Solid Edge part; units mm, degrees
sketch "Sketch1" plane through (0, 0, 0) normal (0, -1, 0) x (1, 0, 0)
  line L0 (-7.5, 10.5) -> (0, 10.5)
  line L1 (0, 10.5) -> (0, 2.95)
  line L2 (-7.5, 2.95) -> (0, 2.95)
  line L3 (-7.5, 10.5) -> (-7.5, 2.95)
  dimension "D1" = 7.5
revolve "RevolvedProtrusion1" add sketch "Sketch1" angle 360 about axis through (0, 0, 0) along (1, 0, 0)
sketch "Sketch2" plane through (-7.5, 0, 0) normal (-1, 0, 0) x (0, -1, 0)
  line L0 (2.9445, -5.1) -> (5.889, 0)
  line L1 (5.889, 0) -> (2.9445, 5.1)
  line L2 (2.9445, 5.1) -> (-2.9445, 5.1)
  line L3 (-2.9445, 5.1) -> (-5.889, 0)
  line L4 (-5.889, 0) -> (-2.9445, -5.1)
  line L5 (-2.9445, -5.1) -> (2.9445, -5.1)
extrude "Cutout1" cut sketch "Sketch2" against normal blind 4.5
chamfer "Fase_2" distance 0.5 angle 45 2 edges at (-7.5, 0, -10.5) (0, 0, -10.5)
hole "Bohrung_1" at (0, -8, 0) direction (-1, 0, 0) diameter 2.2 end up to next
hole "Hole1" at (0, 0, 8) direction (-1, 0, 0) diameter 2.2 end up to next
hole "Hole2" at (0, 0, -8) direction (-1, 0, 0) diameter 2.2 end up to next
hole "Hole3" at (0, 8, 0) direction (-1, 0, 0) diameter 2.2 end up to next
hole "Bohrung_5" at (0, -8, 0) direction (-1, 0, 0) diameter 5.5 depth 2
hole "Hole4" at (0, 0, 8) direction (-1, 0, 0) diameter 5.5 depth 2
hole "Hole5" at (0, 8, 0) direction (-1, 0, 0) diameter 5.5 depth 2
hole "Hole6" at (0, 0, -8) direction (-1, 0, 0) diameter 5.5 depth 2
Part model, mm, in its own coordinate system. A direction names the side the tool comes from. Coordinates: 2 decimals unless noted, no trailing zeros. Write each loop counter-clockwise with the first axis right and the second up, starting at its lowest first coordinate (ties: lowest second). Pieces come first, ordered by that corner, then holes.
Item 1: Pin check, flat tips, straight feed: pin 1 (5 mm diameter, centred on y = 0, z = 8, fed in from +X); pin 2 (1.5 mm diameter, centred on x = -5.5, y = 5.5, fed in from +Z); pin 3 (2 mm diameter, centred on y = 0, z = -8, fed in from -X); pin 4 (4 mm diameter, centred on x = -1.5, z = 5, fed in from -Y). Stop position of each tip, or through.
Item 2: Probe line 1 (Y direction, x = -0.8, z = 0); line 2 (Y direction, x = -6.5, z = -0.25). List the from-to ranges inside material, lowest first.
Item 3: Which spindle directions (+Z, -Z, +X, -X, +Y, -Y) get a long thin tool onto all of the face, cutting with end or side? Do faces 1 (the face through (-7.5, -5, -2)), 2 (the face through (-1.01, 0.1, 5.25)), 3 (the face through (-5.281, 4.396, 2.586)). Say none if no direction does.
Item 4: Slice it at B-B (x = -1). Write the cut outline in (y, z), and give its area (3 significant figures).
Item 5: Slice it at A-A (x = -3.5). Write the cut outline in (y, z).
Results found:
1. pin 1: stops at x = -2
1. pin 2: stops at z = 9.36
1. pin 3: passes through
1. pin 4: stops at y = -10.06
2. line 1: y = -5.25 to -2.95, 2.95 to 5.25
2. line 2: y = -10.5 to -9.07, -6.93 to -5.74, 5.74 to 6.93, 9.07 to 10.5
3. face 1: +Z, -Z, -X, +Y, -Y
3. face 2: +X
3. face 3: -X
4. outline: (-10.42, -1.31) arc R10.5 ccw to (-1.31, -10.42) arc R2.75 cw (long way) to (1.31, -10.42) arc R10.5 ccw to (10.42, -1.31) arc R2.75 cw (long way) to (10.42, 1.31) arc R10.5 ccw to (1.31, 10.42) arc R2.75 cw (long way) to (-1.31, 10.42) arc R10.5 ccw to (-10.42, 1.31) arc R2.75 cw (long way) to start; hole circle Ø5.9 at (0, 0)
4. area: 226 mm2
5. outline: circle Ø21 at (0, 0); hole circle Ø2.2 at (-8, 0); hole (-5.89, 0) - (-2.94, -5.1) - (2.94, -5.1) - (5.89, 0) - (2.94, 5.1) - (-2.94, 5.1) - close; hole circle Ø2.2 at (0, -8); hole circle Ø2.2 at (0, 8); hole circle Ø2.2 at (8, 0)
